from build123d import *

# Parameters (mm, degrees)
F2_R     = 1.5
F3_R     = 0.2
F4_DEPTH = 5
F6_DEPTH = 0.1


with BuildPart() as f1:
    # F0 (on Top) → F1 (revolve)
    with BuildSketch(Plane.XY):
        Polygon((-1.25, 3.3184025263), (-2.75, 3.3184025263), (-2.75, -1.9315974737), (-1.25, -1.9315974737), (-0.9, -1.9315974737), (-0.9, -1.3815974737), (-1.25, -1.3815974737), align=None)
    revolve(axis=Axis((-2.75, 2.1103734641, 0), (0, 1, 0)))

    # F2
    f2_edges = [f1.edges().sort_by_distance(p)[0] for p in [
        (-4.25, 3.318403, 0),
    ]]
    fillet(f2_edges, radius=F2_R)

    # F3 (on face) → F4 (join)
    with BuildSketch(Plane.XZ.offset(1.9315974737)):
        with Locations((-1.5183771327, 0)):
            Circle(F3_R)
        with Locations((-3.9816228673, 0)):
            Circle(F3_R)
    extrude(amount=F4_DEPTH)


with BuildPart() as f5_1:
    # F5: instance of F1
    add(f1.part.mirror(Plane.YZ))


with BuildPart() as f1_1:
    add(f1.part)

    add(f5_1.part)  # F6 merges F5_1
    # F3 (on face) → F6 (join)
    with BuildSketch(Plane.XZ.offset(1.9315974737)):
        with BuildLine():
            Line((4.0972953202, 0.1), (-0.9027046798, 0.1))
            ThreePointArc((-0.9027046798, 0.1), (-0.9006762936, 0.0500182849), (-0.9, 0))
            Line((-0.9, 0), (4.0972953202, 0))
            Line((4.0972953202, 0), (4.0972953202, 0.1))
        make_face()
    extrude(amount=-F6_DEPTH)


solid = f1_1.part
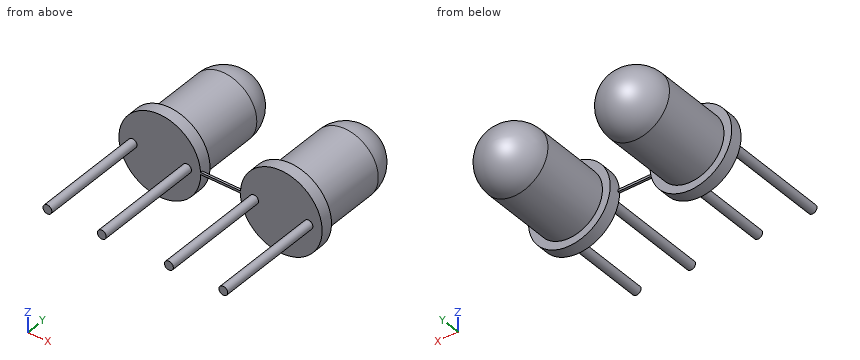
Geometry: final body of the model. Coordinates: model frame, mm. Round coordinates to 2 decimals unless told otherwise and drop trailing zeros. Order: outer loops, then holes, each group sorted by start corner. A loop starts at its lowest first (then second) coordinate and runs counter-clockwise, first axis right, second up.
Q1. Section D-D, the plane x = -0.25. Output: boundary loops of the cut face in (y, z).
Result sheet:
outline: (-1.93, 0) - (-1.83, 0) - (-1.83, 0.1) - (-1.93, 0.1) - close
Q2. Pin query (flat end, axial travel): pin 1 (1 mm diameter, centred on y = -3, z = -1.5, fed in from +X); pin 2 (2 mm diameter, centred on x = -3, z = 1.5, fed in from +Y); pin 3 (1.1 mm diameter, centred on x = 1.5, z = -1, fed in from -Y); pin 4 (2 mm diameter, centred on x = -2, y = -4, fed in from -Z). Return the tip coordinate at first contact, or that it passes through.
Result sheet:
pin 1: passes through
pin 2: stops at y = 3.23
pin 3: stops at y = -1.93
pin 4: stops at z = -0.2
Q3. Section C-C, the plane y = -3.5. Output: boundary loops of the cut face in (x, z).
Result sheet:
outline: circle Ø0.4 at (-3.98, 0); circle Ø0.4 at (-1.52, 0); circle Ø0.4 at (1.52, 0); circle Ø0.4 at (3.98, 0)
Q4. Material intervals for probe 1 along X at (y, z) = (0.5, -0.8); probe 2 along X at (y, z) = (2, 1.15); probe 3 along Y at (x, z) = (1.25, -0.7), sorted ascending.
Result sheet:
probe 1: x = -4.02 to -1.48, 1.48 to 4.02
probe 2: x = -3.7 to -1.8, 1.8 to 3.7
probe 3: y = -1.93 to -1.38
Q5. Section A-A, the plane x = 2.75. Output: boundary loops of the cut face in (y, z), and give its area (3 significant figures).
Result sheet:
outline: (-1.93, -1.85) - (-1.38, -1.85) - (-1.38, -1.5) - (1.82, -1.5) arc R1.5 ccw to (1.82, 1.5) - (-1.38, 1.5) - (-1.38, 1.85) - (-1.93, 1.85) - close
area: 15.2 mm2
Q6. Section B-B, the plane z = 1.05. Output: boundary loops of the cut face in (x, y).
Result sheet:
outline: (-4.27, -1.93) - (-1.23, -1.93) - (-1.23, -1.38) - (-1.68, -1.38) - (-1.68, 1.82) arc R1.07 ccw to (-3.82, 1.82) - (-3.82, -1.38) - (-4.27, -1.38) - close; (1.23, -1.93) - (4.27, -1.93) - (4.27, -1.38) - (3.82, -1.38) - (3.82, 1.82) arc R1.07 ccw to (1.68, 1.82) - (1.68, -1.38) - (1.23, -1.38) - close
